from build123d import *

# Parameters (mm, degrees)
F0_W     = 27.401832
F0_H     = 28.832448
F0_R     = 11.1
F0_R_2   = 4.15
F1_DEPTH = 15
F2_R     = 11.1
F2_R_2   = 4.15
F3_DEPTH = 7


with BuildPart() as f1:
    # F0 (on Front) → F1 (new body)
    with BuildSketch(Plane.XZ):
        Rectangle(F0_W, F0_H)
        Circle(F0_R, mode=Mode.SUBTRACT)
        Circle(F0_R)
        Circle(F0_R_2, mode=Mode.SUBTRACT)
    extrude(amount=F1_DEPTH)

    # F2 (on face) → F3 (cut)
    with BuildSketch(Plane(origin=(0, 0, 0), x_dir=(-1, 0, 0), z_dir=(0, 1, 0))):
        Circle(F2_R)
        Circle(F2_R_2, mode=Mode.SUBTRACT)
    extrude(amount=-F3_DEPTH, mode=Mode.SUBTRACT)


solid = f1.part
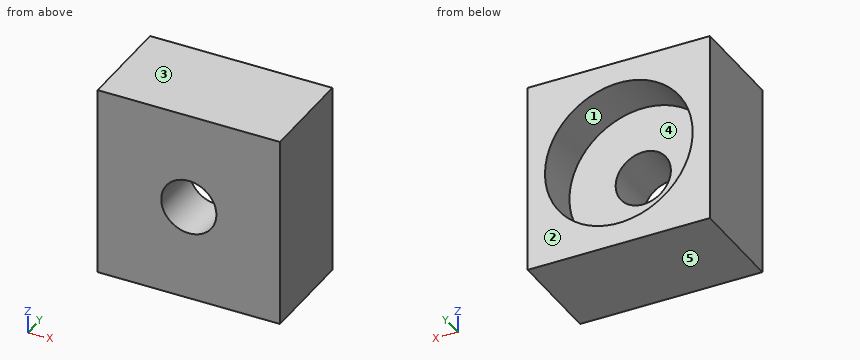
Verification items for the finished model (mm, model axes). Face numbers are marked on the shaded views. A direction names the side the tool comes from. Round coordinates to 2 decimals unless told otherwise and drop trailing zeros. Loops run counter-clockwise (first coordinate to the right, second up) from the corner with the lowest first, then second, coordinate; pieces in that order, holes last. Notation, with made-up numbers: (-14, 42) - (6, 42) arc R29 cw to (6, 78) - close; hole circle Ø10 at (23.5, 56.5). An arc over 180 degrees is marked (long way). Write item = value, one per line.
Q1. Sectioned sample at C-C on y = -1. Record the boundary of the cut face in (x, z), plus the area to 3 significant figures.
Here are the results:
outline = (-13.7, -14.42) - (13.7, -14.42) - (13.7, 14.42) - (-13.7, 14.42) - close; hole circle Ø22.2 at (0, 0)
area = 403 mm^2
Q2. Depth check by flat-ended pin: pin 1 (8 mm diameter, centred on x = -3.5, z = 2, fed in from +Y). Enter the tip coordinate at first touch or a pass-through.
Here are the results:
pin_1 = -7
Q3. Sectioned sample at A-A on z = 0. Record the boundary of the cut face in (x, y), plus the area to 3 significant figures.
Here are the results:
outline = (-13.7, -15) - (-4.15, -15) - (-4.15, -7) - (-11.1, -7) - (-11.1, 0) - (-13.7, 0) - close; (4.15, -15) - (13.7, -15) - (13.7, 0) - (11.1, 0) - (11.1, -7) - (4.15, -7) - close
area = 189 mm^2
Q4. Sectioned sample at B-B on x = 0. Record the boundary of the cut face in (y, z).
Here are the results:
outline = (-15, -14.42) - (0, -14.42) - (0, -11.1) - (-7, -11.1) - (-7, -4.15) - (-15, -4.15) - close; (-15, 4.15) - (-7, 4.15) - (-7, 11.1) - (0, 11.1) - (0, 14.42) - (-15, 14.42) - close
Q5. Tool access check on the marked faces 4 and 5. Record the directions out of +Z, -Z, +X, -X, +Y, -Y that give a thin tool (end or side, any length) a straight path to the whole face; none if there is none.
Here are the results:
face_4 = +Y
face_5 = -Z, +X, -X, +Y, -Y
Q6. Mould release check, pull along Z, two halves, no side actions. Record for the marked faces 1, 2 and 3: +Z half, -Z half, draft (parallel to the pull), parting line (faces both ways), or undercut.
Here are the results:
face_1 = undercut
face_2 = draft
face_3 = +Z half
Q7. Sectioned sample at D-D on x = -7.25. Record the boundary of the cut face in (y, z).
Here are the results:
outline = (-15, -14.42) - (0, -14.42) - (0, -8.41) - (-7, -8.41) - (-7, 8.41) - (0, 8.41) - (0, 14.42) - (-15, 14.42) - close
Q8. Material ranges on L1, parallel to Z at x = 0, y = -4.25; L2, parallel to Y at x = 6.5, z = 0.75; L3, parallel to X at y = -11, z = 0, recorded low to high.
Here are the results:
L1 = -14.42 to -11.1, 11.1 to 14.42
L2 = -15 to -7
L3 = -13.7 to -4.15, 4.15 to 13.7
